```python
from build123d import *

# Parameters (mm, degrees)
SKETCH1_R           = 3
BOSS_EXTRUDE1_DEPTH = 50
SKETCH2_W           = 10
SKETCH2_H           = 148
CUT_EXTRUDE1_DEPTH  = 172.184111412


with BuildPart() as part:
    # Sketch1 → Boss-Extrude1 (new body)
    with BuildSketch(Plane(origin=(0, 0, 0), x_dir=(1, 0, 0), z_dir=(0, 1, 0))):
        with BuildLine():
            Line((0, 0), (0, 148))
            Line((0, 148), (70, 148))
            Line((70, 148), (70, 128))
            ThreePointArc((70, 128), (16, 74), (70, 20))
            Line((70, 20), (70, 0))
            Line((70, 0), (0, 0))
        make_face()
        with Locations(Location((20, 20, 0), (0, 0, 270))):
            Circle(SKETCH1_R, mode=Mode.SUBTRACT)
    extrude(amount=BOSS_EXTRUDE1_DEPTH)

    # Sketch2 → Cut-Extrude1 (cut, through all)
    with BuildSketch(Plane(origin=(0, 50, 0), x_dir=(1, 0, 0), z_dir=(0, 1, 0))):
        with Locations((65, 74)):
            Rectangle(SKETCH2_W, SKETCH2_H)
    extrude(amount=-CUT_EXTRUDE1_DEPTH, mode=Mode.SUBTRACT)


solid = part.part
```
Input: part model. Units: mm. Frame: model coordinates. Coordinates: 2 decimals unless noted, no trailing zeros. Order: outer loops, then holes, each group sorted by start corner. A loop starts at its lowest first (then second) coordinate and runs counter-clockwise, first axis right, second up. Notation, with made-up numbers: (-26, -29) - (28, -29) arc R21 ccw to (28, 10) - close; hole circle Ø7 at (1, -28.75). An arc over 180 degrees is marked (long way). Return JSON: item names as keys, results as strings.
Q1. Cut plane B-B (x = 20). Return loops of the section in (y, z).
The answers:
{"outline": "(0, -148) - (50, -148) - (50, -94.4) - (0, -94.4) - close; (0, -53.6) - (50, -53.6) - (50, -23) - (0, -23) - close; (0, -17) - (50, -17) - (50, 0) - (0, 0) - close"}
Q2. Ray query, probe 1 along X at (y, z) = (11, -20); probe 2 along Z at (x, y) = (21, 10.5); probe 3 along Z at (x, y) = (36, 25.5). Return the intervals inside material, ascending.
The answers:
{"probe 1": "x = 0 to 17, 23 to 60", "probe 2": "z = -148 to -96.69, -51.31 to -22.83, -17.17 to 0", "probe 3": "z = -148 to -115.95, -32.05 to 0"}
Q3. Cut plane D-D (z = -30). Return loops of the section in (x, y).
The answers:
{"outline": "(0, 0) - (38.7, 0) - (38.7, 50) - (0, 50) - close"}
Q4. Cut plane C-C (z = -114). Return loops of the section in (x, y), then the cut area to 3 significant figures.
The answers:
{"outline": "(0, 0) - (33.72, 0) - (33.72, 50) - (0, 50) - close", "area": "1,690 mm2"}
Q5. Draft query along X for faces 1 (the cylindrical face through (16.01, 24.65, -75.05)), 2 (the cylindrical face through (18.2, 24.6, -22.4)), 3 (the flat face through (10, 0, -75)), 4 (the flat face through (0, 25, -73)). Return one class per face: +X half, -X half, draft (parallel to the pull), parting line (faces both ways), or undercut.
The answers:
{"face 1": "+X half", "face 2": "undercut", "face 3": "draft", "face 4": "-X half"}
Q6. Cut plane A-A (y = 9). Return loops of the section in (x, z).
The answers:
{"outline": "(0, -148) - (60, -148) - (60, -127.07) arc R54 cw to (60, -20.93) - (60, 0) - (0, 0) - close; hole circle Ø6 at (20, -20)"}
